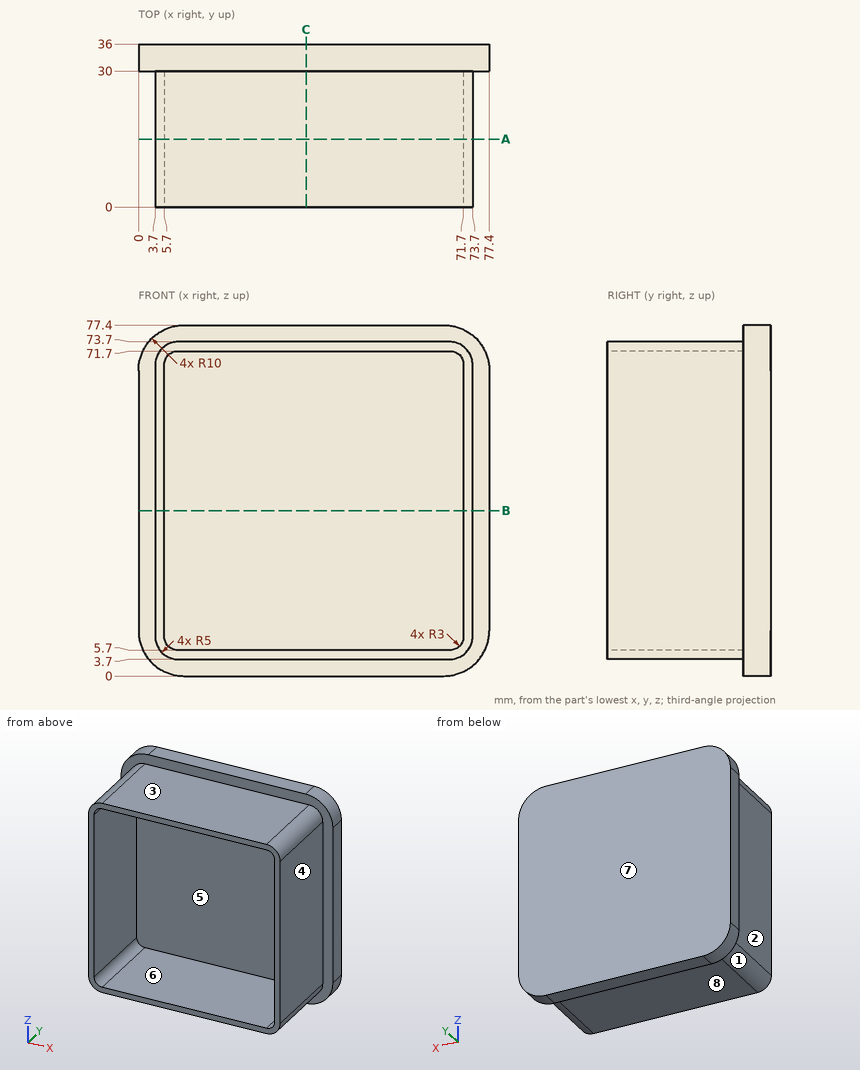
Geometry: see drawing. Coordinates: mm, zero at the bounding-box minimum. A direction names the side the tool comes from. Round coordinates to 2 decimals unless told otherwise and drop trailing zeros. Write each loop counter-clockwise with the first axis right and the second up, starting at its lowest first coordinate (ties: lowest second). Pieces come first, ordered by that corner, then holes.
1) Contact query for flat-ended pins moving along their axis: P1, Ø12, axis at x = 25.5, y = 32, coming from the -Z side; P2, Ø4, axis at y = 6.5, z = 37, coming from the -X side; P3, Ø5, axis at y = 25.5, z = 69.5, coming from the +X side; P4, Ø20, axis at x = 33.5, z = 47.5, coming from the -Y side. Output: stop coordinate, or through.
2) Cut plane A-A (y = 15). Return the cut outline in (x, z).
3) Cut plane B-B (z = 36.5). Return the cut outline in (x, y).
4) Draft query along Z for the marked faces 5, 6, 7 and 8. Return one class per face: pulls with the +Z half, pulls with the -Z half, needs draft (parallel to the pull), parting line crosses it, or undercut.
5) Ray query, L1, parallel to Z at x = 34, y = 20.5; L2, parallel to Y at x = 56.5, z = 6. Return the intervals inside material, ascending.
6) Reachability of the marked faces 1, 2, 3 and 4 from +Z, -Z, +X, -X, +Y, -Y: full face, straight path, thin tool, end or side. Return the list, or none.
7) Cut plane C-C (x = 37). Return the cut outline in (y, z).
Geometry says:
1. P1: stops at z = 0
1. P2: stops at x = 3.7
1. P3: stops at x = 73.7
1. P4: stops at y = 30
2. outline: (3.7, 8.7) arc R5 ccw to (8.7, 3.7) - (68.7, 3.7) arc R5 ccw to (73.7, 8.7) - (73.7, 68.7) arc R5 ccw to (68.7, 73.7) - (8.7, 73.7) arc R5 ccw to (3.7, 68.7) - close; hole (5.7, 8.7) arc R3 ccw to (8.7, 5.7) - (68.7, 5.7) arc R3 ccw to (71.7, 8.7) - (71.7, 68.7) arc R3 ccw to (68.7, 71.7) - (8.7, 71.7) arc R3 ccw to (5.7, 68.7) - close
3. outline: (0, 30) - (3.7, 30) - (3.7, 0) - (5.7, 0) - (5.7, 30) - (71.7, 30) - (71.7, 0) - (73.7, 0) - (73.7, 30) - (77.4, 30) - (77.4, 36) - (0, 36) - close
4. face 5: undercut
4. face 6: undercut
4. face 7: needs draft
4. face 8: pulls with the -Z half
5. L1: z = 3.7 to 5.7, 71.7 to 73.7
5. L2: y = 30 to 36
6. face 1: -Z, -X, -Y
6. face 2: +Z, -Z, -X, -Y
6. face 3: +Z, +X, -X, -Y
6. face 4: +Z, -Z, +X, -Y
7. outline: (0, 3.7) - (30, 3.7) - (30, 0) - (36, 0) - (36, 77.4) - (30, 77.4) - (30, 73.7) - (0, 73.7) - (0, 71.7) - (30, 71.7) - (30, 5.7) - (0, 5.7) - close
